Part model, mm, in its own coordinate system. Face numbers are marked on the shaded views. A direction names the side the tool comes from. Round coordinates to 2 decimals unless told otherwise and drop trailing zeros. Loops run counter-clockwise (first coordinate to the right, second up) from the corner with the lowest first, then second, coordinate; pieces in that order, holes last. Notation, with made-up numbers: M -33,56.25 L -26,56.25 A13 cw -26,60.25 Z; hole C -7.75,-25 d1. An arc over 180 degrees is marked long. Write each question's results on one line, items separated by ' | '.
Autodesk Inventor part; units mm, degrees
ref_plane "YZ Plane" through (0, 0, 0) normal (1, 0, 0) x (0, 1, 0)
ref_plane "XZ Plane" through (0, 0, 0) normal (0, 1, 0) x (-1, 0, 0)
ref_plane "XY Plane" through (0, 0, 0) normal (0, 0, 1) x (1, 0, 0)
sketch "スケッチ1" plane through (0, 0, 0) normal (1, 0, 0) x (0, 1, 0)
  point P0 (0, 0)
sketch "スケッチ2" plane through (0, 0, 0) normal (1, 0, 0) x (0, 1, 0)
  circle A0 centre (0, 0) radius 28.4
  dimension "d0" = 56.8
extrude "押し出し1" add sketch "スケッチ2" along normal blind 6
sketch "スケッチ3" plane through (6, 0, 0) normal (1, 0, 0) x (0, 0, -1)
  circle A0 centre (0, 0) radius 12
  dimension "d3" = 24
extrude "押し出し2" add sketch "スケッチ3" along normal blind 20.4
hole "穴2" at (26.4, 0, 0) direction (-1, 0, 0) diameter 8 end through all
sketch "スケッチ6" plane through (26.4, 0, 0) normal (1, 0, 0) x (0, 0, -1)
  line L0 (0, -5) -> (-1, -5)
  line L1 (-1, -5) -> (-1, -3)
  line L2 (-1, -5) -> (1, -5) construction
  line L3 (-1, -3) -> (1, -3)
  line L4 (1, -3) -> (1, -5)
  line L5 (1, -5) -> (0, -5)
  point P0 (0, 0)
  dimension "d32" = 5
  dimension "d33" = 1
  dimension "d35" = 2
  dimension "d36" = 90
  dimension "d37" = 2
  dimension "d38" = 90
  dimension "d39" = 2
  dimension "d40" = 90
extrude "押し出し5" cut sketch "スケッチ6" against normal blind 26.4
sketch "スケッチ7" plane through (0, 0, 0) normal (-1, 0, 0) x (0, 0, 1)
  circle A0 centre (0, 0) radius 23.75
  line L0 (0, -23.75) -> (-20.5681, -11.875)
  line L1 (-20.5681, -11.875) -> (-20.5681, 11.875)
  line L2 (-20.5681, 11.875) -> (0, 23.75)
  line L3 (0, 23.75) -> (20.5681, 11.875)
  line L4 (20.5681, 11.875) -> (20.5681, -11.875)
  line L5 (20.5681, -11.875) -> (0, -23.75)
  dimension "d43" = 47.5
hole "穴3" at (0, 11.875, 20.5681) at (0, 23.75, 0) at (0, -11.875, 20.5681) at (0, -23.75, 0) at (0, -11.875, -20.5681) at (0, 11.875, -20.5681) direction (1, 0, 0) diameter 5.2 end through all
properties part number "10mmkethub18025"
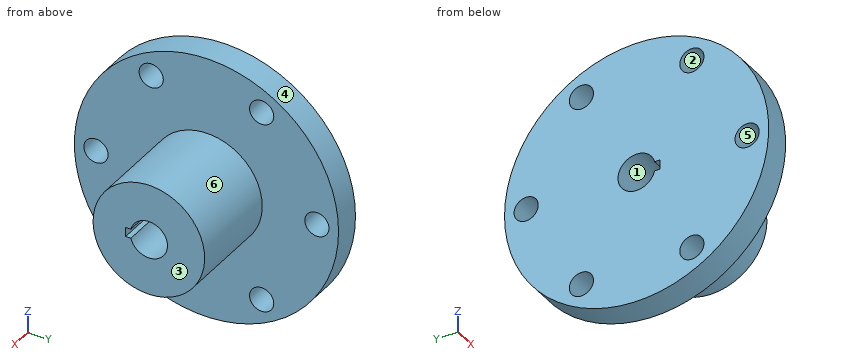
Item 1: Drop flat-ended pins along their axis: P1, Ø4.5, axis at y = -23.75, z = 0, coming from the -X side; P2, Ø6, axis at y = 11.88, z = 20.57, coming from the +X side; P3, Ø10, axis at x = 4.5, y = 20.5, coming from the +Z side; P4, Ø2, axis at x = 10, z = -0.5, coming from the +Y side. Give the stop position or say it passes through.
Filled sheet:
P1: through | P2: x = 6 | P3: z = 23.8 | P4: y = 12
Item 2: Band-saw the part on B-B on y = 0. Give the cut face in (x, z).
Filled sheet:
outline: M 0,-28.4 L 6,-28.4 L 6,-12 L 26.4,-12 L 26.4,-4 L 0,-4 Z; M 0,4 L 26.4,4 L 26.4,12 L 6,12 L 6,28.4 L 0,28.4 Z
Item 3: Two-plate mould, pull along Y, no slides. Class the marked faces 1, 2, 3 and 4: +Y half, -Y half, draft (parallel to the pull), parting line (faces both ways), or undercut.
Filled sheet:
face 1: undercut | face 2: undercut | face 3: draft | face 4: parting line
Item 4: Wall check: L1, parallel to X at y = -18.5, z = 18; L2, parallel to Z at x = 4.5, y = 1; L3, parallel to Y at x = 23.75, z = 2.5. Give the ranges that are in metal, low to high.
Filled sheet:
L1: 0 to 6 | L2: -28.38 to -3.87, 3.87 to 28.38 | L3: -11.74 to -3.12, 3.12 to 11.74
Item 5: Band-saw the part on C-C on x = 15.75. Give the cut face in (y, z), and give its area (3 significant figures).
Filled sheet:
outline: C 0,0 d24; hole M -5,-1 L -3.87,-1 A4 ccw long -3.87,1 L -5,1 Z | area: 400 mm^2
Item 6: Which spindle directions (+Z, -Z, +X, -X, +Y, -Y) get a long thin tool onto all of the face, cutting with end or side? Do the marked faces 5 and 6. Say none if no direction does.
Filled sheet:
face 5: +X, -X | face 6: +X
Item 7: Band-saw the part on A-A on z = 0. Give the cut face in (x, y).
Filled sheet:
outline: M 0,-28.4 L 6,-28.4 L 6,-26.35 L 0,-26.35 Z; M 0,-21.15 L 6,-21.15 L 6,-12 L 26.4,-12 L 26.4,-5 L 0,-5 Z; M 0,4 L 26.4,4 L 26.4,12 L 6,12 L 6,21.15 L 0,21.15 Z; M 0,26.35 L 6,26.35 L 6,28.4 L 0,28.4 Z
Item 8: Band-saw the part on D-D on z = -22. Give the cut face in (x, y).
Filled sheet:
outline: M 0,-17.96 L 6,-17.96 L 6,-14.05 L 0,-14.05 Z; M 0,-9.7 L 6,-9.7 L 6,9.7 L 0,9.7 Z; M 0,14.05 L 6,14.05 L 6,17.96 L 0,17.96 Z
